Input: dimensioned drawing with shaded views. Units: mm. Origin: part minimum x, y, z. A direction names the side the tool comes from. Give positions to 0.01 mm unless a question says otherwise; leave off trailing zeros. Write each loop counter-clockwise with the first axis right and the second up, starting at its lowest first coordinate (ties: lowest second). Pieces come first, ordered by that corner, then holes.
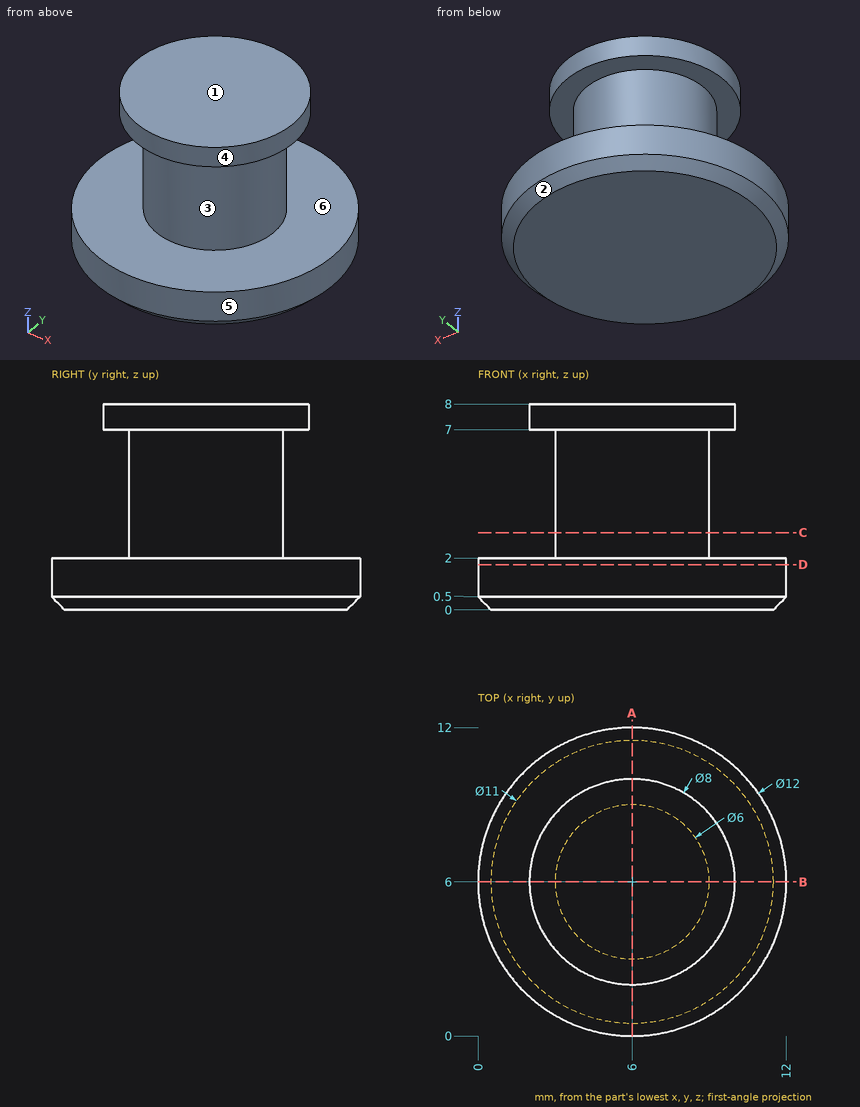
1. Contact query for flat-ended pins moving along their axis: P1, Ø2, axis at y = 7.5, z = 1.5, coming from the +X side; P2, Ø4, axis at x = 10, z = 6.5, coming from the -Y side; P3, Ø2, axis at x = 6, z = 5, coming from the +Y side. Output: stop coordinate, or through.
2. Access query for the marked faces 5 and 6. Directions: +Z, -Z, +X, -X, +Y, -Y. A direction counts if a zero-diameter tool reaches every point of the face in a straight line with its end or side. Return the directions, or none.
3. Mould query, pull axis Z, two halves, no side actions, for the marked faces 1, 2, 3 and 4. Classes: +Z half, -Z half, draft (parallel to the pull), parting line (faces both ways), or undercut.
4. Cut plane A-A, the plane x = 6. Return the cut outline in (y, z).
5. Cut plane C-C, the plane z = 3. Return the cut outline in (x, y).
6. Cut plane D-D, the plane z = 1.75. Return the cut outline in (x, y).
7. Line query: L1, parallel to Z at x = 5.25, y = 2.75; L2, parallel to Z at x = 2, y = 7.5; L3, parallel to X at y = 5.5, z = 4. Output: solid intervals per line, ascending.
Response values:
1. P1: stops at x = 11.98
1. P2: stops at y = 2.57
1. P3: stops at y = 9
2. face 5: +Z, -Z
2. face 6: none
3. face 1: +Z half
3. face 2: -Z half
3. face 3: undercut
3. face 4: draft
4. outline: (0, 0.5) - (0.5, 0) - (11.5, 0) - (12, 0.5) - (12, 2) - (9, 2) - (9, 7) - (10, 7) - (10, 8) - (2, 8) - (2, 7) - (3, 7) - (3, 2) - (0, 2) - close
5. outline: circle Ø6 at (6, 6)
6. outline: circle Ø12 at (6, 6)
7. L1: z = 0 to 2, 7 to 8
7. L2: z = 0 to 2
7. L3: x = 3.04 to 8.96
